Can you work these out from the model? Positions are in its coordinate system, mm. A direction names the side the tool comes from. Coordinates: 2 decimals unless noted, no trailing zeros. Order: outer loops, then holes, each group sorted by start corner. A loop starts at its lowest first (then second) coordinate and runs counter-clockwise, first axis right, second up. Notation, with made-up numbers: M -27.5,20 L -19.5,20 A22 ccw -19.5,34 Z; hole C 57.25,9.25 d7. An arc over 180 degrees is marked long. Answer as CSV lines item,"result". Start each with the question number.
1. If we section it at B-B (z = 17): List the corners of the cut face in (x, y) for me.
2. Will these pins go through, and if not, where does the flat tip stop? pin 1 (4 mm diameter, centred on x = -6, y = 18, fed in from -Z); pin 2 (6 mm diameter, centred on x = 0, z = 16, fed in from +Y); pin 3 (1 mm diameter, centred on x = 6, y = 10, fed in from -Z).
3. I need wall thicknesses on line 1 along Z through (x, y) = (-1, 5); line 2 along Z through (x, y) = (0.5, 4.5); line 3 along X through (y, z) = (9, 0). Which ranges of each line are inside material? Lowest first, please. Write a range as from..to.
4. If we section it at D-D (z = -5): List the corners of the cut face in (x, y) for me, plus the area to 3 significant figures.
5. On a 3-axis mill with a long thin cutter (end or side, diameter ignored), from which of +Z, -Z, +X, -X, +Y, -Y can I reach the whole of each face in a straight line? I mean faces 4 (the face through (-10.74, 21.31, -2.38)), 5 (the face through (-0.2, 0, 4.4)). Say none if no direction works.
6. If we section it at A-A (x = 0): List the corners of the cut face in (y, z) for me.
7. If we mould it in two halves opening along X, with no side actions, what happens to faces 1 (the face through (0, 4, -21)), 2 (the face through (-7, 8, 9)), 3 (the face through (9.097, 4.056, -12.233))? For each: released by +X, released by -X, zero draft, split by the parting line, or undercut.
8. If we section it at C-C (x = 12): List the corners of the cut face in (y, z) for me, plus the area to 3 significant figures.
```python
from build123d import *

# Parameters (mm, degrees)
EXTRUDE_1_DEPTH          = 8
SKETCH_2_R               = 4
CUT_EXTRUDE_1_DEPTH      = 28.018512172
SKETCH_3_R               = 2.4
CUT_EXTRUDE_2_DEPTH      = 8
PATTERN_CIRCULAR_2_COUNT = 8
SKETCH_4_R               = 11
EXTRUDE_2_DEPTH          = 27
SKETCH_5_R               = 4
CUT_EXTRUDE_3_DEPTH      = 44.48562981


with BuildPart() as part:
    # 草图1 → 凸台-拉伸1 (new body)
    with BuildSketch(Plane(origin=(0, 0, 0), x_dir=(1, 0, 0), z_dir=(0, 1, 0))):
        with BuildLine():
            Line((-15, 14.696938457), (-15, -14.696938457))
            ThreePointArc((-15, -14.696938457), (0, -21), (15, -14.696938457))
            Line((15, -14.696938457), (15, 14.696938457))
            ThreePointArc((15, 14.696938457), (0, 21), (-15, 14.696938457))
        make_face()
    extrude(amount=EXTRUDE_1_DEPTH)

    # 草图2 → 切除-拉伸1 (cut, through all)
    with BuildSketch(Plane(origin=(0, 8, 0), x_dir=(1, 0, 0), z_dir=(0, 1, 0))):
        with Locations(Location((0, 0, 0), (0, 0, 270))):
            Circle(SKETCH_2_R)
    extrude(amount=-CUT_EXTRUDE_1_DEPTH, mode=Mode.SUBTRACT)

    # 草图3 → 切除-拉伸2 (cut)
    with BuildSketch(Plane(origin=(0, 8, 0), x_dir=(1, 0, 0), z_dir=(0, 1, 0))):
        with Locations(Location((-11.313708499, 11.313708499, 0), (0, 0, 270))):
            Circle(SKETCH_3_R)
    cut_extrude_2 = extrude(amount=-CUT_EXTRUDE_2_DEPTH, mode=Mode.SUBTRACT)

    # 阵列(圆周)2: 切除-拉伸2 ×8 about axis, 2 skipped
    pattern_circular_2_axis = Axis((0, 8, 0), (0, 1, 0))
    add([cut_extrude_2.rotate(pattern_circular_2_axis, i * 360 / PATTERN_CIRCULAR_2_COUNT) for i in range(1, PATTERN_CIRCULAR_2_COUNT) if i not in (1, 5)], mode=Mode.SUBTRACT)

    # 草图4 → 凸台-拉伸2 (add)
    with BuildSketch(Plane(origin=(0, 8, 0), x_dir=(1, 0, 0), z_dir=(0, 1, 0))):
        with Locations(Location((0, 0, 0), (0, 0, 270))):
            Circle(SKETCH_4_R)
    extrude(amount=EXTRUDE_2_DEPTH)

    # 草图5 → 切除-拉伸3 (cut, through all)
    with BuildSketch(Plane(origin=(0, 35, 0), x_dir=(1, 0, 0), z_dir=(0, 1, 0))):
        with Locations(Location((0, 0, 0), (0, 0, 270))):
            Circle(SKETCH_5_R)
    extrude(amount=-CUT_EXTRUDE_3_DEPTH, mode=Mode.SUBTRACT)


solid = part.part
```
Solved:
1,outline,"M -12.33,0 L -2.18,0 L -2.18,8 L -12.33,8 Z; M 2.18,0 L 12.33,0 L 12.33,8 L 2.18,8 Z"
2,pin 1,"z = -10.25"
2,pin 2,"y = 8"
2,pin 3,"z = -9.53"
3,line 1,"-20.98..-18.18, -13.82..-3.87, 3.87..13.82, 18.18..20.98"
3,line 2,"-20.99..-18.35, -13.65..-3.97, 3.97..13.65, 18.35..20.99"
3,line 3,"-11..-4, 4..11"
4,outline,"M -15,0 L 15,0 L 15,8 L 9.8,8 L 9.8,35 L -9.8,35 L -9.8,8 L -15,8 Z"
4,area,"769 mm²"
5,face 4,"+Y"
5,face 5,"+Z, -Z, +X, -X, -Y"
6,outline,"M 0,-21 L 8,-21 L 8,-18.4 L 0,-18.4 Z; M 0,-13.6 L 8,-13.6 L 8,-11 L 35,-11 L 35,-4 L 0,-4 Z; M 0,4 L 35,4 L 35,11 L 8,11 L 8,13.6 L 0,13.6 Z; M 0,18.4 L 8,18.4 L 8,21 L 0,21 Z"
7,face 1,"split by the parting line"
7,face 2,"zero draft"
7,face 3,"undercut"
8,outline,"M 0,-17.23 L 8,-17.23 L 8,-13.61 L 0,-13.61 Z; M 0,-9.01 L 8,-9.01 L 8,9.01 L 0,9.01 Z; M 0,13.61 L 8,13.61 L 8,17.23 L 0,17.23 Z"
8,area,"202 mm²"
